Check sheet for the modelled part. Datum: model origin and axes. Units: mm. A direction names the side the tool comes from. Round coordinates to 2 decimals unless told otherwise and drop trailing zeros. Loops run counter-clockwise (first coordinate to the right, second up) from the corner with the lowest first, then second, coordinate; pieces in that order, holes last. Notation, with made-up numbers: (89.25, 22.25) - (113.25, 22.25) arc R21 cw to (113.25, 45.25) - close; hole circle Ø9 at (-10.75, 14.5). An arc over 180 degrees is marked (long way). Put each result on its own line as item: value.
```python
from build123d import *

# Parameters (mm, degrees)
POCKET_DEPTH = 2.54


with BuildPart() as part:
    # Sketch → Revolution (revolve)
    with BuildSketch(Plane.YZ):
        Polygon((0, 0), (0, 3.75), (0.45, 3.75), (2.2, 2), (9.751739, 2), (10, 1.57), (10, 0), align=None)
    revolve(axis=Axis((0, 0, 0), (0, 1, 0)))

    # Sketch001 → Pocket (cut)
    with BuildSketch(Plane(origin=(0, 0, 0), x_dir=(0, 0, -1), z_dir=(0, -1, 0))):
        Polygon((-1.905, 0.35), (-0.35, 0.35), (-0.35, 1.905), (0.35, 1.905), (0.35, 0.35), (1.905, 0.35), (1.905, -0.35), (0.35, -0.35), (0.35, -1.905), (-0.35, -1.905), (-0.35, -0.35), (-1.905, -0.35), align=None)
    extrude(amount=-POCKET_DEPTH, mode=Mode.SUBTRACT)


solid = part.part
```
Item 1: Section check B-B on z = 0. Enter the section's corners in (x, y) (3 decimals).
Filled sheet:
outline: (-3.75, 0) - (-1.905, 0) - (-1.905, 2.54) - (1.905, 2.54) - (1.905, 0) - (3.75, 0) - (3.75, 0.45) - (2, 2.2) - (2, 9.752) - (1.57, 10) - (-1.57, 10) - (-2, 9.752) - (-2, 2.2) - (-3.75, 0.45) - close
Item 2: Thickness scan on line 1 (X direction, y = 2.5, z = -1.5); line 2 (Z direction, x = 1, y = 1.75); line 3 (Y direction, x = 2.5, z = 2.5). Record the ranges inside material, lowest first. Write a range as from..to.
Filled sheet:
line 1: -1.32..-0.35, 0.35..1.32
line 2: -2.24..-0.35, 0.35..2.24
line 3: 0..0.66
Item 3: Section check A-A on y = 1. Enter the section's corners in (x, z) (3 decimals).
Filled sheet:
outline: circle Ø6.4 at (0, 0); hole (-1.905, -0.35) - (-0.35, -0.35) - (-0.35, -1.905) - (0.35, -1.905) - (0.35, -0.35) - (1.905, -0.35) - (1.905, 0.35) - (0.35, 0.35) - (0.35, 1.905) - (-0.35, 1.905) - (-0.35, 0.35) - (-1.905, 0.35) - close
Item 4: Go/stop test with flat-tipped pins: pin 1 (1.2 mm diameter, centred on x = 1.5, y = 0.5, fed in from +Z); pin 2 (0.8 mm diameter, centred on y = 1.5, z = 1, fed in from -X); pin 3 (0.5 mm diameter, centred on x = -1.5, y = 1, fed in from +Z). Record where each tip stops, or that it passes through.
Filled sheet:
pin 1: z = 3.64
pin 2: x = -2.95
pin 3: z = 3.13
Item 5: Section check C-C on x = 0. Enter the section's corners in (y, z) (3 decimals), then the cut area to 3 significant figures.
Filled sheet:
outline: (0, -3.75) - (0.45, -3.75) - (2.2, -2) - (9.752, -2) - (10, -1.57) - (10, 1.57) - (9.752, 2) - (2.2, 2) - (0.45, 3.75) - (0, 3.75) - (0, 1.905) - (2.54, 1.905) - (2.54, -1.905) - (0, -1.905) - close
area: 34.9 mm²
Item 6: Section check D-D on y = 6.25. Enter the section's corners in (x, z), then the cut area to 3 significant figures.
Filled sheet:
outline: circle Ø4 at (0, 0)
area: 12.6 mm²
Item 7: Tool access check on faces 5 (the cylindrical face through (-2, 6, 0)), 6 (the flat face through (0, 10, 0)), 7 (the flat face through (0.35, 1, -1)). Record the directions out of +Z, -Z, +X, -X, +Y, -Y that give a thin tool (end or side, any length) a straight path to the whole face; none if there is none.
Filled sheet:
face 5: +Y
face 6: +Z, -Z, +X, -X, +Y
face 7: -Y
Item 8: Release check for a two-part mould opening along X. For faces 1 (the flat face through (-1, 0, -1)), 2 (the flat face through (1, 1, -0.35)), 3 (the cylindrical face through (0.165, 0.228, -3.746)), 4 (the flat face through (0, 2.54, 0)) record: +X half, -X half, draft (parallel to the pull), parting line (faces both ways), or undercut.
Filled sheet:
face 1: draft
face 2: undercut
face 3: parting line
face 4: undercut
